The figure shows three views and two pictorial views of one solid part (mm, origin at its lowest corner). Answer the questions. A direction names the side the tool comes from. Round coordinates to 2 decimals unless told otherwise and drop trailing zeros. Order: outer loops, then holes, each group sorted by start corner. A loop starts at its lowest first (then second) coordinate and runs counter-clockwise, first axis right, second up. Notation, with made-up numbers: (-2.75, 9.5) -> (47.25, 9.5) arc R32 ccw to (47.25, 39.5) -> close; hole circle Ø2 at (69, -2.75). An arc over 180 degrees is marked (long way). Answer in a Markdown table with one row per item. Add a question column.
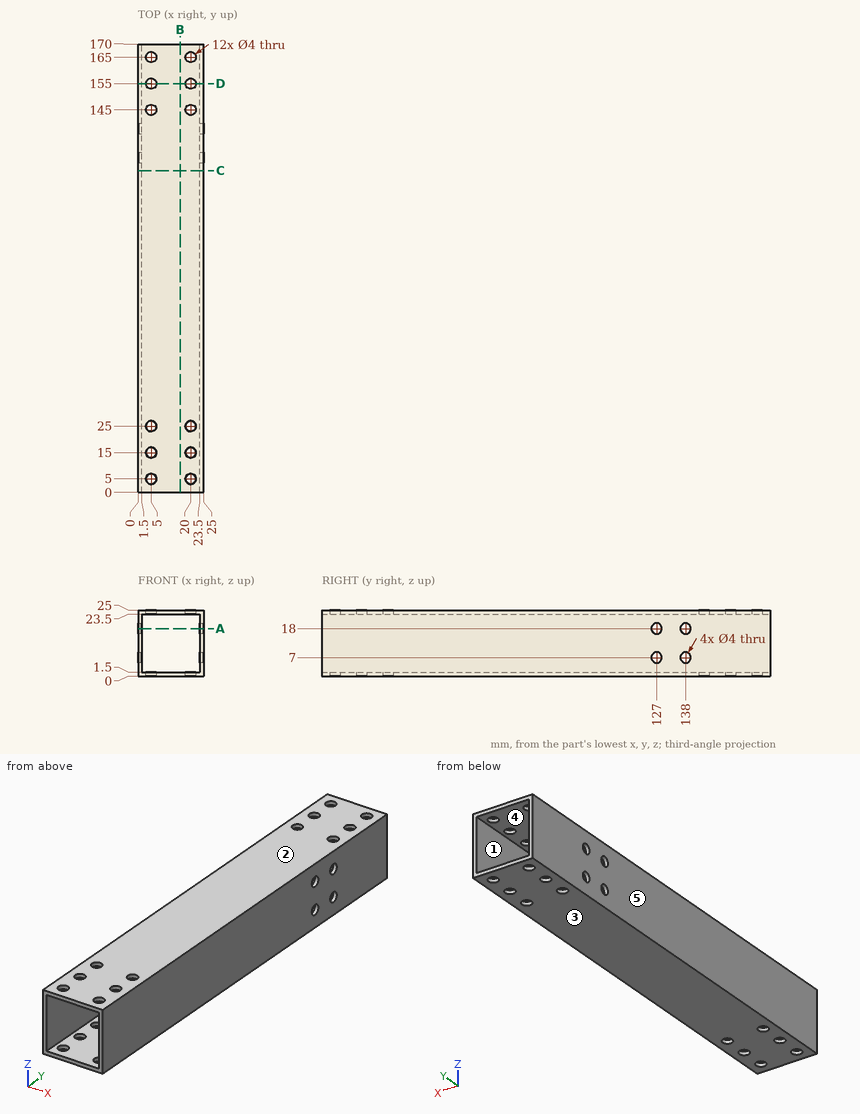
1. The mould has two halves that part along Z. Classify the marked faces 3, 4 and 5: released by +Z, released by -Z, zero draft, split by the parting line, or undercut.
2. The part is cut by section B-B (x = 16). Give the vertices of the cut face in (y, z).
3. The part is cut by section D-D (y = 155). Give the vertices of the cut face in (x, z).
4. For the marked faces 1 and 2, determine the directions among +Z, -Z, +X, -X, +Y, -Y from which every point of the face is accessible in a straight line to the end or side of a thin tool.
5. The part is cut by section C-C (y = 122). Give the vertices of the cut face in (x, z), then the cut area to 3 significant figures.
6. The part is cut by section A-A (z = 18). Give the vertices of the cut face in (x, y).
7. Straight lines are drawn through the part: line 1 along X through (y, z) = (25, 24.65); line 2 along X through (y, z) = (141.5, 12.5). For each, find the intervals that lie inside material, in ascending order.
Report:
| question | item | result |
|---|---|---|
| 1 | face 3 | released by -Z |
| 1 | face 4 | undercut |
| 1 | face 5 | zero draft |
| 2 | outline | (0, 0) -> (170, 0) -> (170, 1.5) -> (0, 1.5) -> close; (0, 23.5) -> (170, 23.5) -> (170, 25) -> (0, 25) -> close |
| 3 | outline | (0, 0) -> (3, 0) -> (3, 1.5) -> (1.5, 1.5) -> (1.5, 23.5) -> (3, 23.5) -> (3, 25) -> (0, 25) -> close; (7, 0) -> (18, 0) -> (18, 1.5) -> (7, 1.5) -> close; (7, 23.5) -> (18, 23.5) -> (18, 25) -> (7, 25) -> close; (22, 0) -> (25, 0) -> (25, 25) -> (22, 25) -> (22, 23.5) -> (23.5, 23.5) -> (23.5, 1.5) -> (22, 1.5) -> close |
| 4 | face 1 | +Y, -Y |
| 4 | face 2 | +Z, +X, -X, +Y, -Y |
| 5 | outline | (0, 0) -> (25, 0) -> (25, 25) -> (0, 25) -> close; hole (1.5, 1.5) -> (23.5, 1.5) -> (23.5, 23.5) -> (1.5, 23.5) -> close |
| 5 | area | 141 mm^2 |
| 6 | outline | (0, 0) -> (1.5, 0) -> (1.5, 125) -> (0, 125) -> close; (0, 129) -> (1.5, 129) -> (1.5, 136) -> (0, 136) -> close; (0, 140) -> (1.5, 140) -> (1.5, 170) -> (0, 170) -> close; (23.5, 0) -> (25, 0) -> (25, 125) -> (23.5, 125) -> close; (23.5, 129) -> (25, 129) -> (25, 136) -> (23.5, 136) -> close; (23.5, 140) -> (25, 140) -> (25, 170) -> (23.5, 170) -> close |
| 7 | line 1 | x = 0 to 3, 7 to 18, 22 to 25 |
| 7 | line 2 | x = 0 to 1.5, 23.5 to 25 |
